Part model, mm, in its own coordinate system. A direction names the side the tool comes from. Round coordinates to 2 decimals unless told otherwise and drop trailing zeros. Loops run counter-clockwise (first coordinate to the right, second up) from the corner with the lowest first, then second, coordinate; pieces in that order, holes last. Notation, with made-up numbers: M -17,35 L -5,35 A31 cw -5,59 Z; hole C 27.25,-24.5 d11. An arc over 180 degrees is marked long. Put each result on its own line as item: value. Start each with the question number.
1) Which spindle directions (+Z, -Z, +X, -X, +Y, -Y) get a long thin tool onto all of the face, cutting with end or side? Do faces 1 (the flat face through (26, -1, 4)), 2 (the cylindrical face through (12.1, 45, 5.5)), 3 (the flat face through (0, 1, 0)), 4 (the flat face through (-20, -40, 2)), 5 (the flat face through (-20, 47, 3)). Say none if no direction does.
2) Pull direction Y, two halves, no side cores. Call faces 6 (the flat face through (-25, 4, 8)), 7 (the flat face through (0, 1, 2)), 8 (the cylindrical face through (18, 38.5, 5)), 9 (the flat face through (-20, 49, 1)): +Y half, -Y half, draft (parallel to the pull), parting line (faces both ways), or undercut.
3) Probe line 1 along Y through (x, z) = (20, 4.1); line 2 along Y through (x, z) = (-3, 7); line 3 along Y through (x, z) = (19, 5.75). List the from-to ranges inside material, lowest first.
4) Slice it at C-C on x = -20. Give the cut face in (y, z), then the cut area to 3 significant figures.
5) Slice it at B-B on y = 47.5. Give the cut face in (x, z), then the cut area to 3 significant figures.
6) Slice it at A-A on z = 4. State how many separate pieces and enclosed holes the cut face has, then the cut area to 3 significant figures.
7) Drop flat-ended pins along their axis: pin 1 Ø2 at (x, y) = (20, -40) entering from +Z; pin 2 Ø0.6 at (x, y) = (0.5, -45) entering from +Z; pin 3 Ø2.5 at (y, z) = (47.5, 1.5) entering from +X. Give the stop position or say it passes through.
8) Slice it at D-D on x = -13.5. Give the cut face in (y, z), then the cut area to 3 significant figures.
```python
from build123d import *

# Parameters (mm, degrees)
SKETCH1_W           = 52
SKETCH1_H           = 92
SKETCH1_W_2         = 48
SKETCH1_H_2         = 88
EXTRUDE_THIN1_DEPTH = 8
SKETCH2_W           = 48
SKETCH2_H           = 88
BOSS_EXTRUDE1_DEPTH = 2
FILLET1_R           = 5
SKETCH3_R           = 2.5
SKETCH3_R_2         = 1.1
BOSS_EXTRUDE2_DEPTH = 6
SKETCH4_R           = 2.5
CUT_EXTRUDE1_DEPTH  = 10
SKETCH5_W           = 5
SKETCH5_H           = 2
CUT_EXTRUDE2_DEPTH  = 10
FILLET2_R           = 1
SKETCH6_W           = 3
SKETCH6_H           = 3
BOSS_EXTRUDE3_DEPTH = 3
SKETCH7_R           = 1
CUT_EXTRUDE3_DEPTH  = 3


with BuildPart() as part:
    # Sketch1 → Extrude-Thin1 (new body)
    with BuildSketch(Plane.XY):
        Rectangle(SKETCH1_W, SKETCH1_H)
        Rectangle(SKETCH1_W_2, SKETCH1_H_2, mode=Mode.SUBTRACT)
    extrude(amount=EXTRUDE_THIN1_DEPTH)

    # Sketch2 → Boss-Extrude1 (add)
    with BuildSketch(Plane.XY):
        Rectangle(SKETCH2_W, SKETCH2_H)
    extrude(amount=BOSS_EXTRUDE1_DEPTH)

    # Fillet1
    fillet1_edges = [part.edges().sort_by_distance(p)[0] for p in [
        (-26, 46, 4),
        (26, 46, 4),
        (26, -46, 4),
        (-26, -46, 4),
    ]]
    fillet(fillet1_edges, radius=FILLET1_R)

    # Sketch3 → Boss-Extrude2 (add)
    # profile 1 of 4: a face of its own
    with BuildSketch(Plane.XY.offset(2)):
        with Locations((-20, 40)):
            Circle(SKETCH3_R)
        with Locations((-20, 40)):
            Circle(SKETCH3_R_2, mode=Mode.SUBTRACT)
    # profile 2 of 4: a face of its own
    with BuildSketch(Plane.XY.offset(2)):
        with Locations((-20, -40)):
            Circle(SKETCH3_R)
        with Locations((-20, -40)):
            Circle(SKETCH3_R_2, mode=Mode.SUBTRACT)
    # profile 3 of 4: a face of its own
    with BuildSketch(Plane.XY.offset(2)):
        with Locations((20, -40)):
            Circle(SKETCH3_R)
        with Locations((20, -40)):
            Circle(SKETCH3_R_2, mode=Mode.SUBTRACT)
    # profile 4 of 4: a face of its own
    with BuildSketch(Plane.XY.offset(2)):
        with Locations((20, 40)):
            Circle(SKETCH3_R)
        with Locations((20, 40)):
            Circle(SKETCH3_R_2, mode=Mode.SUBTRACT)
    extrude(amount=BOSS_EXTRUDE2_DEPTH)

    # Sketch4 → Cut-Extrude1 (cut)
    with BuildSketch(Plane(origin=(0, 46, 0), x_dir=(1, 0, 0), z_dir=(0, 1, 0))):
        with Locations((12, -8)):
            Circle(SKETCH4_R)
    extrude(amount=-CUT_EXTRUDE1_DEPTH, mode=Mode.SUBTRACT)

    # Sketch5 → Cut-Extrude2 (cut)
    with BuildSketch(Plane.XZ.offset(46)):
        with Locations((0, 8)):
            Rectangle(SKETCH5_W, SKETCH5_H)
    extrude(amount=-CUT_EXTRUDE2_DEPTH, mode=Mode.SUBTRACT)

    # Fillet2
    fillet2_edges = [part.edges().sort_by_distance(p)[0] for p in [
        (-2.5, -45, 7),
        (2.5, -45, 7),
    ]]
    fillet(fillet2_edges, radius=FILLET2_R - 0.0001)  # a hair under: the kernel refuses the full size

    # Sketch6 → Boss-Extrude3 (add)
    with BuildSketch(Plane(origin=(0, 46, 0), x_dir=(1, 0, 0), z_dir=(0, 1, 0))):
        with Locations((-19.5, -1.5)):
            Rectangle(SKETCH6_W, SKETCH6_H)
    extrude(amount=BOSS_EXTRUDE3_DEPTH)

    # Sketch7 → Cut-Extrude3 (cut)
    with BuildSketch(Plane.ZY.offset(21)):
        with Locations(Location((1.5, 47.5, 0), (0, 0, 270))):
            Circle(SKETCH7_R)
    extrude(amount=-CUT_EXTRUDE3_DEPTH, mode=Mode.SUBTRACT)


solid = part.part
```
Recorded:
1. face 1: +Z, -Z, +X, +Y, -Y
1. face 2: +Z, +Y
1. face 3: -Z, +X, -X, +Y, -Y
1. face 4: +Z
1. face 5: +Z, +X, -X, +Y
2. face 6: draft
2. face 7: undercut
2. face 8: undercut
2. face 9: +Y half
3. line 1: y = -46 to -44, -42.5 to -41.1, -38.9 to -37.5, 37.5 to 38.9, 41.1 to 42.5, 44 to 46
3. line 2: y = -46 to -44, 44 to 46
3. line 3: y = -46 to -44, -42.29 to -40.46, -39.54 to -37.71, 37.71 to 39.54, 40.46 to 42.29, 44 to 46
4. outline: M -46,0 L 49,0 L 49,3 L 46,3 L 46,8 L 44,8 L 44,2 L 42.5,2 L 42.5,8 L 41.1,8 L 41.1,2 L 38.9,2 L 38.9,8 L 37.5,8 L 37.5,2 L -37.5,2 L -37.5,8 L -38.9,8 L -38.9,2 L -41.1,2 L -41.1,8 L -42.5,8 L -42.5,2 L -44,2 L -44,8 L -46,8 Z; hole C 47.5,1.5 d2
4. area: 247 mm2
5. outline: M -21,0 L -18,0 L -18,0.5 L -21,0.5 Z; M -21,2.5 L -18,2.5 L -18,3 L -21,3 Z
5. area: 3.00 mm2
6. separate pieces: 5
6. enclosed holes: 5
6. area: 602 mm2
7. pin 1: stops at z = 2
7. pin 2: stops at z = 7
7. pin 3: stops at x = -18
8. outline: M -46,0 L 46,0 L 46,8 L 44,8 L 44,2 L -44,2 L -44,8 L -46,8 Z
8. area: 208 mm2
